from build123d import *

# Parameters (mm, degrees)
SKETCH1_R                       = 12.7
SKETCH1_R_2                     = 4.7625
BOSS_EXTRUDE1_DEPTH             = 2.8575
F_6_32_TAPPED_HOLE1_D           = 2.7051
CUT_EXTRUDE1_DEPTH              = 3.96875
F_9_64_0_14063_DIAMETER_HOLE1_D = 3.572002
FILLET1_R                       = 0.635


with BuildPart() as part:
    # Sketch1 → Boss-Extrude1 (new, symmetric)
    with BuildSketch(Plane.XY):
        Circle(SKETCH1_R)
        Circle(SKETCH1_R_2, mode=Mode.SUBTRACT)
    extrude(amount=BOSS_EXTRUDE1_DEPTH, both=True)

    # #6-32 Tapped Hole1 (through all)
    with Locations(Plane.XY.offset(2.8575)):
        with Locations((5.612660076, 5.612660076), (5.612660076, -5.612660076), (-5.612660076, -5.612660076), (-5.612660076, 5.612660076)):
            Hole(F_6_32_TAPPED_HOLE1_D / 2)

    # Sketch5 → Cut-Extrude1 (cut)
    with BuildSketch(Plane.XY.offset(2.8575)):
        with BuildLine():
            Line((9.779, 2.921), (12.305192125, 3.142013173))
            ThreePointArc((12.305192125, 3.142013173), (12.7, 0), (12.305192125, -3.142013173))
            Line((12.305192125, -3.142013173), (9.779, -2.921))
            ThreePointArc((9.779, -2.921), (6.858, 0), (9.779, 2.921))
        make_face()
        with BuildLine():
            Line((2.921, -9.779), (3.142013173, -12.305192125))
            ThreePointArc((3.142013173, -12.305192125), (0, -12.7), (-3.142013173, -12.305192125))
            Line((-3.142013173, -12.305192125), (-2.921, -9.779))
            ThreePointArc((-2.921, -9.779), (0, -6.858), (2.921, -9.779))
        make_face()
        with BuildLine():
            Line((-9.779, -2.921), (-12.305192125, -3.142013173))
            ThreePointArc((-12.305192125, -3.142013173), (-12.7, 0), (-12.305192125, 3.142013173))
            Line((-12.305192125, 3.142013173), (-9.779, 2.921))
            ThreePointArc((-9.779, 2.921), (-6.858, 0), (-9.779, -2.921))
        make_face()
        with BuildLine():
            Line((-2.921, 9.779), (-3.142013173, 12.305192125))
            ThreePointArc((-3.142013173, 12.305192125), (0, 12.7), (3.142013173, 12.305192125))
            Line((3.142013173, 12.305192125), (2.921, 9.779))
            ThreePointArc((2.921, 9.779), (0, 6.858), (-2.921, 9.779))
        make_face()
    extrude(amount=-CUT_EXTRUDE1_DEPTH, mode=Mode.SUBTRACT)

    # 9/64 (0.14063) Diameter Hole1 (through all)
    with Locations(Plane.XY.offset(-1.11125)):
        with Locations((0, 9.779), (-9.779, 0), (0, -9.779), (9.779, 0)):
            Hole(F_9_64_0_14063_DIAMETER_HOLE1_D / 2)

    # Fillet1
    fillet1_edges = [part.edges().sort_by_distance(p)[0] for p in [
        (12.305192125, 3.142013173, 0.873125),
        (12.305192125, -3.142013173, 0.873125),
        (3.142013173, -12.305192125, 0.873125),
        (-3.142013173, -12.305192125, 0.873125),
        (-12.305192125, -3.142013173, 0.873125),
        (-12.305192125, 3.142013173, 0.873125),
        (-3.142013173, 12.305192125, 0.873125),
        (3.142013173, 12.305192125, 0.873125),
    ]]
    fillet(fillet1_edges, radius=FILLET1_R)


solid = part.part
Can you work these out from the model? Positions are in its coordinate system, mm. A direction names the side the tool comes from. Give positions to 0.01 mm unless a question says otherwise; leave off trailing zeros. Order: outer loops, then holes, each group sorted by start corner. A loop starts at its lowest first (then second) coordinate and runs counter-clockwise, first axis right, second up. Notation, with made-up numbers: (-29, 60.25) - (-15, 60.25) arc R8 cw to (-15, 66.25) - close; hole circle Ø8 at (-8.5, 75). An arc over 180 degrees is marked (long way). Write each question's results on one line, items separated by ' | '.
1) I'm going to push flat-ended pins straight in: pin 1 Ø7.5 at (x, y) = (0, 0) entering from -Z; pin 2 Ø1 at (x, z) = (3.5, -2) entering from -Y; pin 3 Ø1.8 at (x, y) = (11, 1.5) entering from +Z. Where does each tip first touch, or does it pass through?
Final values:
pin 1: passes through | pin 2: stops at y = -12.34 | pin 3: stops at z = -1.11
2) Suppose I cut it at D-D, the plane z = -1.65. Give the number of separate pieces and of enclosed holes in the cut face, then the cut area to 3 significant figures.
Final values:
separate pieces: 1 | enclosed holes: 9 | area: 372 mm^2
3) If we mould it in two halves opening along Y, with no side actions, what happens to faces 5 (the face through (-6, 0, 2.858)), 6 (the face through (-3, -10.7, 0.9)), 7 (the face through (12, 0, -1.111)), 8 (the face through (3, 10.7, 0.9))? For each: pulls with the +Y half, pulls with the -Y half, needs draft (parallel to the pull), parting line crosses it, or undercut.
Final values:
face 5: needs draft | face 6: pulls with the -Y half | face 7: undercut | face 8: pulls with the +Y half
4) Suppose I cut it at A-A, the plane y = 0. Write out the boundary of the cut face in (x, z) (1 decimal).
Final values:
outline: (-12.7, -2.9) - (-11.6, -2.9) - (-11.6, -1.1) - (-12.7, -1.1) - close; (-8, -2.9) - (-4.8, -2.9) - (-4.8, 2.9) - (-6.9, 2.9) - (-6.9, -1.1) - (-8, -1.1) - close; (4.8, -2.9) - (8, -2.9) - (8, -1.1) - (6.9, -1.1) - (6.9, 2.9) - (4.8, 2.9) - close; (11.6, -2.9) - (12.7, -2.9) - (12.7, -1.1) - (11.6, -1.1) - close
5) Please list where these lines run through material, in increasing order: line 1 along Y through (x, z) = (0, -1.95) (1 decimal); line 2 along Y through (x, z) = (0.75, -2.1); line 3 along Y through (x, z) = (0, 1.3). Write a range as [from, to].
Final values:
line 1: y = [-12.7, -11.6], [-8, -4.8], [4.8, 8], [11.6, 12.7] | line 2: y = [-12.68, -11.4], [-8.16, -4.7], [4.7, 8.16], [11.4, 12.68] | line 3: y = [-6.86, -4.76], [4.76, 6.86]
6) Suppose I cut it at C-C, the plane y = -6.25. Write out the boundary of the cut face in (x, z).
Final values:
outline: (-11.06, -2.86) - (-6.81, -2.86) - (-6.81, 2.86) - (-11.06, 2.86) - close; (-4.42, -2.86) - (4.42, -2.86) - (4.42, 2.86) - (-4.42, 2.86) - close; (6.81, -2.86) - (11.06, -2.86) - (11.06, 2.86) - (6.81, 2.86) - close
7) On a 3-axis mill with a long thin cutter (end or side, diameter ignored), from which of +Z, -Z, +X, -X, +Y, -Y can I reach the whole of each face in a straight line? I mean faces 1 (the face through (0, -12, -1.111)), 2 (the face through (10.646, 2.997, 0.901)), 3 (the face through (4.89, -4.47, -0.04)), 4 (the face through (-10.646, -2.997, 0.901)). Say none if no direction works.
Final values:
face 1: +Z, -Y | face 2: +Z, +X | face 3: +Z, -Z | face 4: +Z, -X
